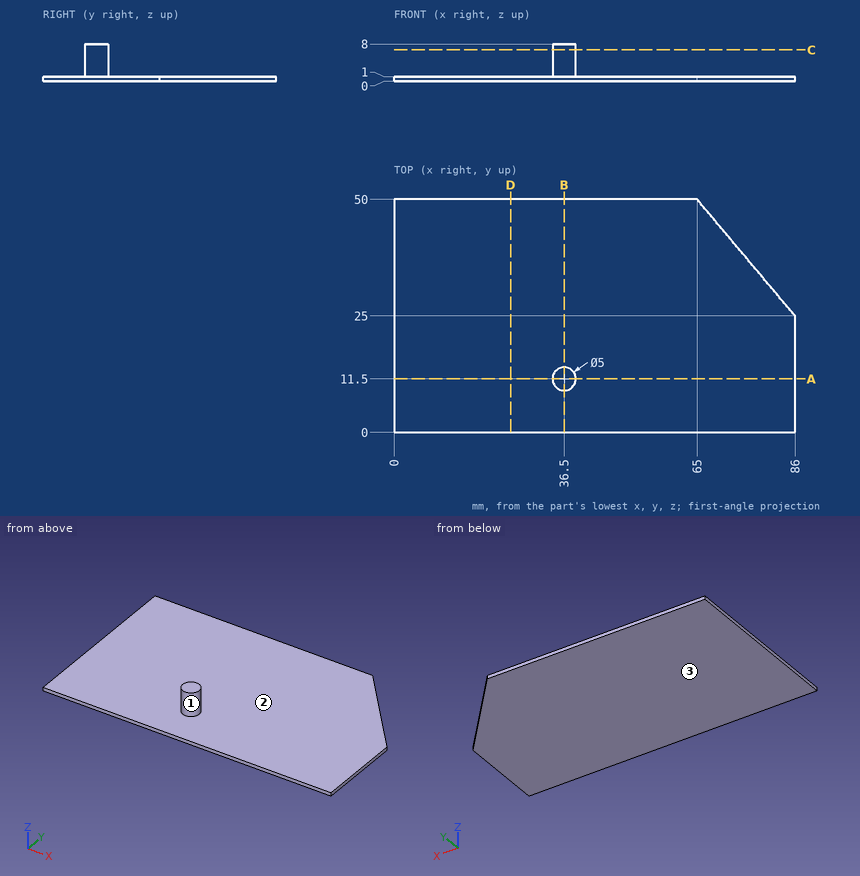
Check sheet for the drawn part. Datum: minimum x, y, z corner. Units: mm. Round coordinates to 2 decimals unless told otherwise and drop trailing zeros. Write each loop counter-clockwise with the first axis right and the second up, starting at its lowest first coordinate (ties: lowest second). Pieces come first, ordered by that corner, then holes. Notation, with made-up numbers: (44.5, 72) -> (92.5, 72) arc R37 cw to (92.5, 109) -> close; hole circle Ø11 at (-21, 31.5). An arc over 180 degrees is marked (long way). Write each question's results on one line, items separated by ' | '. Start each with the question number.
1. Depth check by flat-ended pin: P1, Ø1.5, axis at x = 70, y = 26.5, coming from the +Z side; P2, Ø6, axis at x = 18, y = 8.5, coming from the -Z side. Enter the tip coordinate at first touch or a pass-through.
2. Draft check along Z on the marked faces 1, 2 and 3. Enter one of: +Z half, -Z half, draft (parallel to the pull), parting line (faces both ways), or undercut.
3. Cross-section at A-A (y = 11.5). Enter the section's corners in (x, z).
4. Cross-section at B-B (x = 36.5). Enter the section's corners in (y, z), then the cut area to 3 significant figures.
5. Cross-section at C-C (z = 6.75). Enter the section's corners in (x, y).
6. Cross-section at D-D (x = 25). Enter the section's corners in (y, z).
7. Material ranges on probe 1 along Z at (x, y) = (49, 11.5); probe 2 along X at (y, z) = (10.5, 5.25); probe 3 along Y at (x, z) = (37, 6.5), recorded low to high. Write a range as from..to.
Solutions:
1) P1: stops at z = 1 | P2: stops at z = 0
2) face 1: draft | face 2: +Z half | face 3: -Z half
3) outline: (0, 0) -> (86, 0) -> (86, 1) -> (39, 1) -> (39, 8) -> (34, 8) -> (34, 1) -> (0, 1) -> close
4) outline: (0, 0) -> (50, 0) -> (50, 1) -> (14, 1) -> (14, 8) -> (9, 8) -> (9, 1) -> (0, 1) -> close | area: 85.0 mm2
5) outline: circle Ø5 at (36.5, 11.5)
6) outline: (0, 0) -> (50, 0) -> (50, 1) -> (0, 1) -> close
7) probe 1: z = 0..1 | probe 2: x = 34.21..38.79 | probe 3: y = 9.05..13.95
